For this review, take the finished solid that the model builds, in its own axes (mm). A direction names the side the tool comes from. Coordinates: 2 decimals unless noted, no trailing zeros. Write each loop counter-clockwise with the first axis right and the second up, starting at its lowest first coordinate (ties: lowest second). Pieces come first, ordered by that corner, then holes. Notation, with made-up numbers: M 37,86.5 L 81,86.5 A34 cw 81,124.5 Z; hole C 77,46.5 d9. An arc over 180 degrees is marked long. One line per question, with ' | ' between items.
from build123d import *

# Parameters (mm, degrees)
BOSS_EXTRUDE1_START = 4
BOSS_EXTRUDE1_DEPTH = 2.5


with BuildPart() as part:
    # Sketch1 → Revolve1 (revolve)
    with BuildSketch(Plane.XY):
        Polygon((0, 0), (0, 12.8), (2.9, 12.8), (2.9, 22.8), (6, 22.8), (6, 21), (5.4, 21), (5.4, 16), (4.6, 16), (4.6, 6), (1.5, 6), (1.5, 0), align=None)
    revolve(axis=Axis((0, 0, 0), (0, 1, 0)))

    # Sketch2 → Boss-Extrude1 (add)
    with BuildSketch(Plane.XZ.offset(-21).offset(BOSS_EXTRUDE1_START)):
        Polygon((8.082903769, 0), (4.041451884, 7), (-4.041451884, 7), (-8.082903769, 0), (-4.041451884, -7), (4.041451884, -7), align=None)
    extrude(amount=BOSS_EXTRUDE1_DEPTH)

    # Sketch3 → Cut-Revolve1 (revolve, cut)
    with BuildSketch(Plane.XY):
        with BuildLine():
            Line((-8.082903769, 16.7), (-8.082903769, 17))
            Line((-8.082903769, 17), (-7, 17))
            ThreePointArc((-7, 17), (-7.561845302, 16.923613695), (-8.082903769, 16.7))
        make_face()
        with BuildLine():
            Line((-8.082903769, 14.8), (-8.082903769, 14.5))
            Line((-8.082903769, 14.5), (-7, 14.5))
            ThreePointArc((-7, 14.5), (-7.561845302, 14.576386305), (-8.082903769, 14.8))
        make_face()
    revolve(axis=Axis((0, 14.5, 0), (0, 1, 0)), mode=Mode.SUBTRACT)


solid = part.part
1) The part is to be moulded in two halves that separate along Z. For faces 6 (the flat face through (6.034, 15.768, -3.549)), 7 (the flat face through (0, 14.5, 0)), 8 (the cylindrical face through (-6, 22, 0)), say which applies: +Z half, -Z half, draft (parallel to the pull), parting line (faces both ways), or undercut.
Responses:
face 6: -Z half | face 7: undercut | face 8: parting line
2) Insertion check: pin 1 Ø1.5 at (y, z) = (11, 3.5) entering from -X; pin 2 Ø1.5 at (x, y) = (-2.5, 12) entering from -Z; pin 3 Ø1 at (y, z) = (13, 1.5) entering from +X; pin 4 Ø5 at (x, z) = (0, 0) entering from -Y. Each pin has a flat end and moves straight along its axis. Give the tip position at first contact, or say it passes through.
Responses:
pin 1: x = -3.69 | pin 2: z = -4.25 | pin 3: x = 4.49 | pin 4: y = 0
3) Machinability: for faces 1 (the cylindrical face through (-3.65, 10.19, 2.8)), 2 (the flat face through (-3, 22.8, -1)), 3 (the cylindrical face through (-2.9, 13.7, -0.1)), 4 (the flat face through (0, 16, -7)), 5 (the cylindrical face through (-2.9, 19.9, -0.1)), which of the approach directions +Z, -Z, +X, -X, +Y, -Y give a long, thin tool a straight path to every point of the face, cutting with its end or side? Answer none if there is none.
Responses:
face 1: -Y | face 2: +Z, -Z, +X, -X, +Y | face 3: none | face 4: -Z, +X, -X, +Y, -Y | face 5: +Y
4) We need section B-B on y = 16. State the section outline as (x, z) points, then the cut area to 3 significant figures.
Responses:
outline: M -8.08,0 L -4.04,-7 L 4.04,-7 L 8.08,0 L 4.04,7 L -4.04,7 Z | area: 170 mm^2
5) We need section A-A on y = 19.5. State the section outline as (x, z) points, then the cut area to 3 significant figures.
Responses:
outline: C 0,0 d10.8; hole C 0,0 d5.8 | area: 65.2 mm^2
6) We need section C-C on y = 7. State the section outline as (x, z) points.
Responses:
outline: C 0,0 d9.2
7) To check wall thickness, follow line 1 along Y through (x, z) = (-0.75, 2.75); line 2 along Y through (x, z) = (0.75, -1.25); line 3 along Z through (x, y) = (0, 13.55). State the ranges of each line that lie inside material, in increasing order. Write a range as [from, to].
Responses:
line 1: [6, 12.8], [14.5, 17] | line 2: [0, 12.8], [14.5, 17] | line 3: [-4.6, -2.9], [2.9, 4.6]
